Check sheet for the modelled part. Datum: model origin and axes. Units: mm. Face numbers are marked on the shaded views. A direction names the side the tool comes from. Coordinates: 2 decimals unless noted, no trailing zeros. Order: outer loops, then holes, each group sorted by start corner. A loop starts at its lowest first (then second) coordinate and runs counter-clockwise, first axis right, second up.
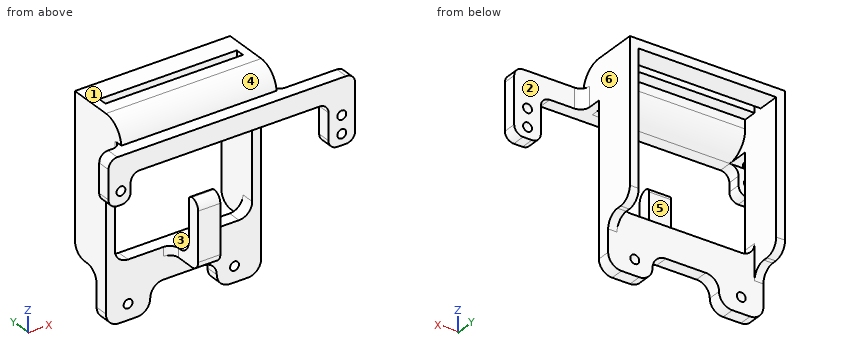
from build123d import *

# Parameters (mm, degrees)
SKETCH_1_W          = 35
SKETCH_1_H          = 35
SKETCH_1_W_2        = 31
SKETCH_1_H_2        = 31
EXTRUDE_1_DEPTH     = 10
EXTRUDE_2_DEPTH     = 5
SKETCH_3_W          = 31
SKETCH_3_H          = 7
CUT_EXTRUDE_1_DEPTH = 3
SKETCH_4_W          = 5
SKETCH_4_H          = 4.5
SKETCH_4_W_2        = 35
SKETCH_4_H_2        = 6
SKETCH_4_R          = 1
SKETCH_4_W_3        = 6
SKETCH_4_H_3        = 10
EXTRUDE_3_DEPTH     = 3
FILLET_2_R          = 2
FILLET_3_R          = 2
SKETCH_5_W          = 5
SKETCH_5_H          = 2
EXTRUDE_4_DEPTH     = 8.3
SKETCH_6_W          = 5
SKETCH_6_H          = 13
EXTRUDE_5_DEPTH     = 3
FILLET_4_R          = 2
FILLET_5_R          = 1
FILLET_6_R          = 2
SKETCH_7_W          = 31
SKETCH_7_H          = 2
CUT_EXTRUDE_2_DEPTH = 10
FILLET_7_R          = 5
SKETCH_8_W          = 35
SKETCH_8_H          = 11
SKETCH_8_R          = 1
EXTRUDE_6_DEPTH     = 3
FILLET_8_R          = 3
FILLET_9_R          = 3
SKETCH_11_W         = 15
SKETCH_11_H         = 6
CUT_EXTRUDE_4_DEPTH = 3
FILLET_START        = -1
FILLET_10_DEPTH     = 4
FILLET_10_2_DEPTH   = 3
FILLET_11_R         = 3


with BuildPart() as part:
    # 草图1 → 凸台-拉伸1 (new body)
    with BuildSketch(Plane(origin=(0, 0, 0), x_dir=(1, 0, 0), z_dir=(0, 1, 0))):
        Rectangle(SKETCH_1_W, SKETCH_1_H)
        Rectangle(SKETCH_1_W_2, SKETCH_1_H_2, mode=Mode.SUBTRACT)
    extrude(amount=EXTRUDE_1_DEPTH)

    # 草图2 → 凸台-拉伸2 (add)
    with BuildSketch(Plane.XZ):
        Polygon((15.5, 8.5), (17.5, 8.5), (17.5, 17.5), (-17.5, 17.5), (-17.5, 8.5), align=None)
    extrude(amount=EXTRUDE_2_DEPTH)

    # 草图3 → 切除-拉伸1 (cut)
    with BuildSketch(Plane(origin=(0, 0, -17.5), x_dir=(-1, 0, 0), z_dir=(0, 0, -1))):
        with Locations((0, 6.5)):
            Rectangle(SKETCH_3_W, SKETCH_3_H)
    extrude(amount=-CUT_EXTRUDE_1_DEPTH, mode=Mode.SUBTRACT)

    # 草图4 → 凸台-拉伸3 (add)
    # profile 1 of 5: a face of its own
    with BuildSketch(Plane.XZ.offset(5)):
        with Locations((-20, 10.75)):
            Rectangle(SKETCH_4_W, SKETCH_4_H)
    # profile 2 of 5: a face of its own
    with BuildSketch(Plane.XZ.offset(5)):
        with Locations((0, 10.75)):
            Rectangle(SKETCH_4_W_2, SKETCH_4_H)
    # profile 3 of 5: a face of its own
    with BuildSketch(Plane.XZ.offset(5)):
        with Locations((-20, 5.5)):
            Rectangle(SKETCH_4_W, SKETCH_4_H_2)
        with Locations(Location((-19.7, 5.46, 0), (0, 0, 270))):
            Circle(SKETCH_4_R, mode=Mode.SUBTRACT)
    # profile 4 of 5: a face of its own
    with BuildSketch(Plane.XZ.offset(5)):
        Polygon((17.5, 13), (17.5, 8.5), (27.1, 8.5), (33.1, 8.5), (33.1, 13), align=None)
    # profile 5 of 5: a face of its own
    with BuildSketch(Plane.XZ.offset(5)):
        with Locations((30.1, 3.5)):
            Rectangle(SKETCH_4_W_3, SKETCH_4_H_3)
        with Locations(Location((30.1, 0.96, 0), (0, 0, 270))):
            Circle(SKETCH_4_R, mode=Mode.SUBTRACT)
        with Locations(Location((30.1, 4.96, 0), (0, 0, 270))):
            Circle(SKETCH_4_R, mode=Mode.SUBTRACT)
    extrude(amount=EXTRUDE_3_DEPTH)

    # 圆角2
    fillet_2_edges = [part.edges().sort_by_distance(p)[0] for p in [
        (-22.5, -6.5, 13),
        (-22.5, -6.5, 2.5),
        (-17.5, -6.5, 2.5),
        (-17.5, -6.5, 8.5),
        (27.1, -6.5, 8.5),
        (27.1, -6.5, -1.5),
        (33.1, -6.5, -1.5),
        (33.1, -6.5, 13),
    ]]
    fillet(fillet_2_edges, radius=FILLET_2_R)

    # 圆角3
    fillet_3_edges = [part.edges().sort_by_distance(p)[0] for p in [
        (17.5, -5, 10.75),
        (-17.5, -5, 10.75),
    ]]
    fillet(fillet_3_edges, radius=FILLET_3_R)

    # 草图5 → 凸台-拉伸4 (add)
    with BuildSketch(Plane.XZ):
        with Locations((0, -16.5)):
            Rectangle(SKETCH_5_W, SKETCH_5_H)
    extrude(amount=EXTRUDE_4_DEPTH)

    # 草图6 → 凸台-拉伸5 (add)
    with BuildSketch(Plane.XZ.offset(8.3)):
        with Locations((0, -9)):
            Rectangle(SKETCH_6_W, SKETCH_6_H)
    extrude(amount=-EXTRUDE_5_DEPTH)

    # 圆角4
    fillet_4_edges = [part.edges().sort_by_distance(p)[0] for p in [
        (0, -8.3, -17.5),
        (0, -8.3, -2.5),
    ]]
    fillet(fillet_4_edges, radius=FILLET_4_R)

    # 圆角5
    fillet_5_edges = [part.edges().sort_by_distance(p)[0] for p in [
        (0, -5.3, -2.5),
    ]]
    fillet(fillet_5_edges, radius=FILLET_5_R - 0.0001)  # a hair under: the kernel refuses the full size

    # 圆角6
    fillet_6_edges = [part.edges().sort_by_distance(p)[0] for p in [
        (2.5, 0, -16.5),
        (-2.5, 0, -16.5),
    ]]
    fillet(fillet_6_edges, radius=FILLET_6_R)

    # 草图7 → 切除-拉伸2 (cut)
    with BuildSketch(Plane(origin=(0, 0, 15.5), x_dir=(-1, 0, 0), z_dir=(0, 0, -1))):
        with Locations((0, 4)):
            Rectangle(SKETCH_7_W, SKETCH_7_H)
    extrude(amount=-CUT_EXTRUDE_2_DEPTH, mode=Mode.SUBTRACT)

    # 圆角7
    # the kernel refuses this fillet: 5 mm, written as the material it takes off along each edge
    with BuildSketch(Plane(origin=(-15.5, 0, 8.5), x_dir=(0, -1, 0), z_dir=(1, 0, 0))) as fillet_7_piece_1:
        with BuildLine():
            CenterArc((FILLET_7_R, -FILLET_7_R), FILLET_7_R, 90, 90)
            Line((0, -FILLET_7_R), (0, 0))
            Line((0, 0), (FILLET_7_R, 0))
        make_face()
    extrude(amount=31, mode=Mode.SUBTRACT)
    with BuildSketch(Plane(origin=(29.937342964, -5, 17.5), x_dir=(0, 0, -1), z_dir=(-1, 0, 0))) as fillet_7_piece_2:
        with BuildLine():
            CenterArc((5, -4.974937186), FILLET_7_R, 95.739170477, 84.260829523)
            Line((0, -4.974937186), (0, 0))
            Line((0, 0), (4.5, 0))
        make_face()
    extrude(amount=59.874685928, mode=Mode.SUBTRACT)

    # 草图8 → 凸台-拉伸6 (add)
    with BuildSketch(Plane(origin=(0, 3, 0), x_dir=(1, 0, 0), z_dir=(0, 1, 0))):
        with Locations((0, 23)):
            Rectangle(SKETCH_8_W, SKETCH_8_H)
        with Locations(Location((11.5, 25, 0), (0, 0, 270))):
            Circle(SKETCH_8_R, mode=Mode.SUBTRACT)
        with Locations(Location((-12.5, 25, 0), (0, 0, 270))):
            Circle(SKETCH_8_R, mode=Mode.SUBTRACT)
    extrude(amount=-EXTRUDE_6_DEPTH)

    # 圆角8
    fillet_8_edges = [part.edges().sort_by_distance(p)[0] for p in [
        (16.5, 3, -17.5),
        (-16.5, 3, -17.5),
        (-17.5, 1.5, -28.5),
        (17.5, 1.5, -28.5),
        (-16.5, 10, -17.5),
        (16.5, 10, -17.5),
    ]]
    fillet(fillet_8_edges, radius=FILLET_8_R)

    # 圆角9
    fillet_9_edges = [part.edges().sort_by_distance(p)[0] for p in [
        (-15.5, 1.5, -15.5),
        (15.5, 1.5, -15.5),
    ]]
    fillet(fillet_9_edges, radius=FILLET_9_R)

    # 草图11 → 切除-拉伸4 (cut)
    with BuildSketch(Plane.XZ):
        with Locations((0, -25.5)):
            Rectangle(SKETCH_11_W, SKETCH_11_H)
    extrude(amount=-CUT_EXTRUDE_4_DEPTH, mode=Mode.SUBTRACT)

    # 圆角10: read off the stored shape, not the designer's step
    # 圆角10 outline → 圆角10 (cut)
    with BuildSketch(Plane(origin=(0, 0, 0), x_dir=(1, 0, 0), z_dir=(0, 1, 0)).offset(FILLET_START)):
        with BuildLine():
            Line((7.5, 28.5), (7.5, 25.5))
            ThreePointArc((7.5, 25.5), (8.378679656, 27.621320344), (10.5, 28.5))
            Line((10.5, 28.5), (7.5, 28.5))
        make_face()
        with BuildLine():
            ThreePointArc((-10.5, 28.5), (-8.378679656, 27.621320344), (-7.5, 25.5))
            Line((-7.5, 25.5), (-7.5, 28.5))
            Line((-7.5, 28.5), (-10.5, 28.5))
        make_face()
    extrude(amount=FILLET_10_DEPTH, mode=Mode.SUBTRACT)

    # Fillet 10 2 outline → Fillet 10 2 (add)
    with BuildSketch(Plane(origin=(0, 0, 0), x_dir=(1, 0, 0), z_dir=(0, 1, 0))):
        with BuildLine():
            Line((-7.5, 22.5), (-4.5, 22.5))
            ThreePointArc((-4.5, 22.5), (-6.621320344, 23.378679656), (-7.5, 25.5))
            Line((-7.5, 25.5), (-7.5, 22.5))
        make_face()
        with BuildLine():
            ThreePointArc((7.5, 25.5), (6.621320344, 23.378679656), (4.5, 22.5))
            Line((4.5, 22.5), (7.5, 22.5))
            Line((7.5, 22.5), (7.5, 25.5))
        make_face()
    extrude(amount=FILLET_10_2_DEPTH)

    # 圆角11
    fillet_11_edges = [part.edges().sort_by_distance(p)[0] for p in [
        (0, -5.3, -15.5),
    ]]
    fillet(fillet_11_edges, radius=FILLET_11_R)


solid = part.part
(1) Cross-section at D-D (x = 24). Enter the section's corners in (y, z), and give its area (3 significant figures).
Filled in:
outline: (-8, 8.5) - (-5, 8.5) - (-5, 13) - (-8, 13) - close
area: 13.5 mm2
(2) Tool access check on the marked faces 1, 2 and 3. Record the directions out of +Z, -Z, +X, -X, +Y, -Y that give a thin tool (end or side, any length) a straight path to the whole face; none if there is none.
Filled in:
face 1: +Z, +X, -X, +Y, -Y
face 2: +Z, -Z, +X, +Y
face 3: +Y
(3) Go/stop test with flat-tipped pins: P1, Ø2.5, axis at x = -19.7, z = 5.46, coming from the -Y side; P2, Ø10, axis at x = 19.5, y = 4.5, coming from the -Z side; P3, Ø3, axis at y = -4.5, z = -7, coming from the -X side. Record where each tip stops, or that it passes through.
Filled in:
P1: stops at y = -8
P2: stops at z = -28.49
P3: stops at x = -2.5
(4) Cross-section at A-A (x = 1.5). Count the separate pieces of the cut face and the enclosed holes in it, and give its area (3 significant figures).
Filled in:
separate pieces: 3
enclosed holes: 0
area: 140 mm2
(5) Release check for a two-part mould opening along Z. For the marked faces 4, 5 and 6 record: +Z half, -Z half, draft (parallel to the pull), parting line (faces both ways), or undercut.
Filled in:
face 4: +Z half
face 5: undercut
face 6: draft
(6) Cross-section at B-B (x = 11.5). Enter the section's corners in (y, z), and give its area (3 significant figures).
Filled in:
outline: (-8, 8.5) - (-5, 8.5) arc R5 ccw to (0, 13.5) - (0, 15.5) - (3, 15.5) - (3, 17.5) - (-0.03, 17.5) arc R5 ccw to (-5, 13) - (-8, 13) - close; (0, -28.5) - (3, -28.5) - (3, -26) - (0, -26) - close; (0, -24) - (3, -24) - (3, -15.5) - (0, -15.5) - close; (5, 15.5) - (10, 15.5) - (10, 17.5) - (5, 17.5) - close
area: 96.9 mm2
(7) Cross-section at C-C (z = -8). Enter the section's corners in (x, y), and give its area (3 significant figures).
Filled in:
outline: (-17.5, 0) - (-15.5, 0) - (-15.5, 10) - (-17.5, 10) - close; (-2.5, -8.3) - (2.5, -8.3) - (2.5, -5.3) - (-2.5, -5.3) - close; (15.5, 0) - (17.5, 0) - (17.5, 10) - (15.5, 10) - close
area: 55.0 mm2
(8) Thickness scan on probe 1 along X at (y, z) = (5, -16.5); probe 2 along X at (y, z) = (-7.35, 0.96); probe 3 along X at (y, z) = (1.35, -25). Record the ranges inside material, lowest first.
Filled in:
probe 1: x = -17.5 to -15.5, 15.5 to 17.5
probe 2: x = 27.1 to 29.1, 31.1 to 33.1
probe 3: x = -17.5 to -13.5, -11.5 to -7.46, 7.46 to 10.5, 12.5 to 17.5
